Source: three-view drawing plus pictorial views. Frame: mm from the lowest corner of the part. A direction names the side the tool comes from. Round coordinates to 2 decimals unless told otherwise and drop trailing zeros. Order: outer loops, then holes, each group sorted by start corner. A loop starts at its lowest first (then second) coordinate and runs counter-clockwise, first axis right, second up. Notation, with made-up numbers: (3, 26) -> (32, 26) arc R23 cw to (32, 57) -> close; hole circle Ø7 at (88, -23.75). An arc over 180 degrees is marked (long way). Answer as CSV lines item,"result".
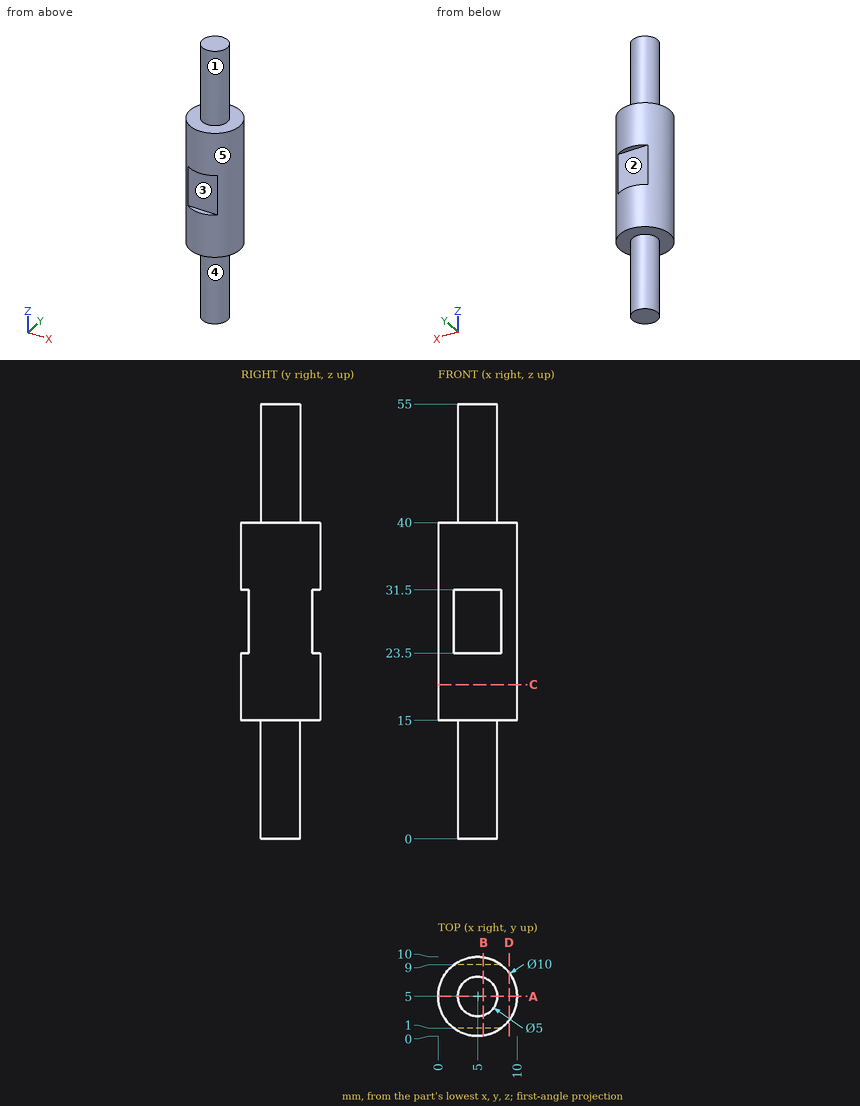
1. Line query: L1, parallel to X at y = 2, z = 17; L2, parallel to Y at x = 9, z = 26; L3, parallel to Z at x = 1.5, y = 2.5. Output: solid intervals per line, ascending. Write a range as [from, to].
Results below:
L1,"[1, 9]"
L2,"[2, 8]"
L3,"[15, 40]"
2. Section query C-C on z = 19.5. Return loops of the section in (x, y), and give its area (3 significant figures).
Results below:
outline,"circle Ø10 at (5, 5)"
area,"78.5 mm2"
3. Section query D-D on x = 9. Return loops of the section in (y, z), and give its area (3 significant figures).
Results below:
outline,"(2, 15) -> (8, 15) -> (8, 40) -> (2, 40) -> close"
area,"150 mm2"
4. Section query B-B on x = 5.75. Return loops of the section in (y, z).
Results below:
outline,"(0.06, 15) -> (2.62, 15) -> (2.62, 0) -> (7.38, 0) -> (7.38, 15) -> (9.94, 15) -> (9.94, 23.5) -> (9, 23.5) -> (9, 31.5) -> (9.94, 31.5) -> (9.94, 40) -> (7.38, 40) -> (7.38, 55) -> (2.62, 55) -> (2.62, 40) -> (0.06, 40) -> (0.06, 31.5) -> (1, 31.5) -> (1, 23.5) -> (0.06, 23.5) -> close"
5. Pin query (flat end, axial travel): pin 1 (1.5 mm diameter, centred on x = 4.5, z = 6.5, fed in from -Y); pin 2 (1.5 mm diameter, centred on y = 8, z = 16.5, fed in from -X); pin 3 (1.5 mm diameter, centred on y = 2.5, z = 22.5, fed in from -X). Return the tip coordinate at first contact, or that it passes through.
Results below:
pin 1,"y = 2.5"
pin 2,"x = 0.53"
pin 3,"x = 0.32"
6. Section query A-A on y = 5. Return loops of the section in (x, z), and give its area (3 significant figures).
Results below:
outline,"(0, 15) -> (2.5, 15) -> (2.5, 0) -> (7.5, 0) -> (7.5, 15) -> (10, 15) -> (10, 40) -> (7.5, 40) -> (7.5, 55) -> (2.5, 55) -> (2.5, 40) -> (0, 40) -> close"
area,"400 mm2"
7. Reachability of the marked faces 4 and 5 from +Z, -Z, +X, -X, +Y, -Y: full face, straight path, thin tool, end or side. Return the list, or none.
Results below:
face 4,"-Z"
face 5,"+Z, -Z"
8. Mould query, pull axis Z, two halves, no side actions, for the marked faces 1, 2 and 3. Classes: released by +Z, released by -Z, zero draft, split by the parting line, or undercut.
Results below:
face 1,"zero draft"
face 2,"undercut"
face 3,"undercut"
